Design review of the part built by this model. Coordinates are the model's own, in mm. Coordinates: 2 decimals unless noted, no trailing zeros. Order: outer loops, then holes, each group sorted by start corner. A loop starts at its lowest first (then second) coordinate and runs counter-clockwise, first axis right, second up. Notation, with made-up numbers: (35.5, -7.5) - (86.5, -7.5) arc R24 cw to (86.5, 12.5) - close; hole circle Ø8 at (87, 44). An arc over 180 degrees is marked (long way). Write item = value, one per line. Start each with the question number.
```python
from build123d import *

# Parameters (mm, degrees)
F1_DEPTH    = 3.175
F3_DEPTH    = 25.4
F4_T1_DEPTH = 21.629832931
F4_T3_DEPTH = 25.208081251
F6_D        = 3.175


# Not quite as in the source:
# - a fillet or chamfer that OpenCascade refuses, or shapes differently, is made with other operations: its cross-section is extruded or revolved along the edge and cut away or added


with BuildPart() as f1:
    # F0 (on Top) → F1 (new body, symmetric)
    with BuildSketch(Plane.XY):
        Polygon((-31.6706262529, 7.0008751936), (-31.4483754337, 0), (29.8926271498, 0), align=None)
    extrude(amount=F1_DEPTH, both=True)

    # F2 (on Front) → F3 (cut)
    with BuildSketch(Plane.XZ):
        Polygon((-32.3509715194, 5.2941306494), (-32.3509715194, 1.5875), (-19.0253787046, 1.5875), (-19.1175676882, 5.2941306494), align=None)
        Polygon((-19.0253787046, -1.5875), (-32.3509715194, -1.5875), (-32.3509715194, -5.2941306494), (-19.1175676882, -5.2941306494), align=None)
    extrude(amount=-F3_DEPTH, mode=Mode.SUBTRACT)

    # F4: fillet of radius 3.81 on 2 edges, made by hand

    # F4_s2 → F4_t1 (cut)
    with BuildSketch(Plane.XY.offset(-10.8149164655)):
        with BuildLine():
            ThreePointArc((-27.7574088475, 0), (-30.4083993967, 1.0735151913), (-31.5654904043, 3.6891080797))
            Line((-31.5654904043, 3.6891080797), (-31.4483754337, 0))
            Line((-31.4483754337, 0), (-27.7574088475, 0))
        make_face()
    extrude(amount=F4_T1_DEPTH, mode=Mode.SUBTRACT)

    # F4_s4 → F4_t3 (cut)
    with BuildSketch(Plane.XY.offset(-12.6040406255)):
        with BuildLine():
            ThreePointArc((-27.2922295058, 6.5029708841), (-30.3048140162, 5.5189587428), (-31.5308036019, 2.5964777998))
            Line((-31.5308036019, 2.5964777998), (-31.6706262529, 7.0008751936))
            Line((-31.6706262529, 7.0008751936), (-27.2922295058, 6.5029708841))
        make_face()
    extrude(amount=F4_T3_DEPTH, mode=Mode.SUBTRACT)

    # F6 (through all)
    with Locations(Plane(origin=(0, 0, -3.175), x_dir=(1, 0, 0), z_dir=(0, 0, -1))):
        with Locations((-27.722722045, -2.71736972)):
            Hole(F6_D / 2)


solid = f1.part
```
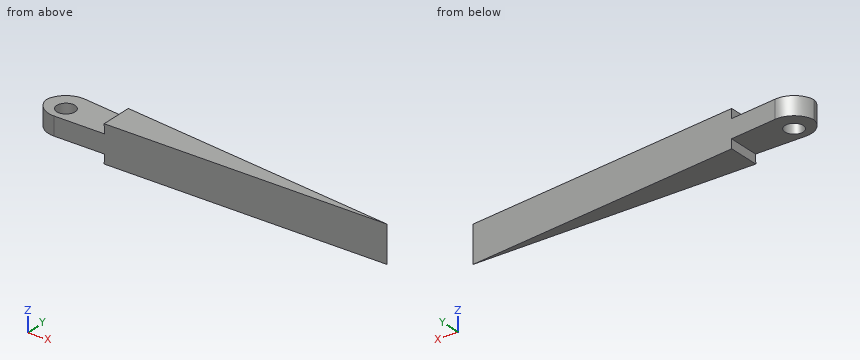
Item 1: Add section D-D on x = -3. Give the boundary of the cut face in (y, z) (1 decimal), plus the area to 3 significant figures.
Item 2: Add section B-B on y = 1.75. Give the boundary of the cut face in (x, z) (1 decimal), plus the area to 3 significant figures.
Item 3: For P1, Ø3.5, axis at x = -25, y = 4, coming from the -Z side; P2, Ø1, axis at x = -1.5, z = 0, coming from the +Y side; P3, Ø2, axis at y = 2.5, z = 0, coming from the -X side; P4, Ø3.5, axis at x = -24, y = 4, coming from the +Z side, all flat-tipped, find the tip position at first contact; note any pin that passes through.
Item 4: For line 1 (Z direction, x = -25.5, y = 2.5); line 2 (Y direction, x = -20, z = -1.25); line 3 (Y direction, x = -18, z = 2.5), list the stretches that pass through material, from the lowest coordinate up.
Item 5: Add section A-A on z = -0.75. Give the boundary of the cut face in (x, y) (1 decimal), plus the area to 3 significant figures.
Item 6: Add section C-C on y = 5. Give the boundary of the cut face in (x, z) (1 decimal), plus the area to 3 significant figures.
Worked out:
q1.outline = (0, -3.2) - (3.7, -3.2) - (3.7, 3.2) - (0, 3.2) - close
q1.area = 23.8 mm2
q2.outline = (-31, -1.6) - (-29, -1.6) - (-29, 1.6) - (-31, 1.6) - close; (-26.5, -1.6) - (-19, -1.6) - (-19.1, -3.2) - (14.5, -3.2) - (14.5, 3.2) - (-19.1, 3.2) - (-19, 1.6) - (-26.5, 1.6) - close
q2.area = 243 mm2
q3.P1 = -1.59
q3.P2 = 3.63
q3.P3 = -31.51
q3.P4 = 1.59
q4.line_1 = -1.59 to 1.59
q4.line_2 = 0 to 5.67
q4.line_3 = 0 to 5.45
q5.outline = (-31.5, 3.1) arc R3.8 ccw to (-27.8, 0) - (29.9, 0) - (-27.3, 6.5) arc R3.8 ccw to start; hole circle Ø3.2 at (-27.7, 2.7)
q5.area = 200 mm2
q6.outline = (-30.8, -1.6) - (-19, -1.6) - (-19.1, -3.2) - (-14.1, -3.2) - (-14.1, 3.2) - (-19.1, 3.2) - (-19, 1.6) - (-30.8, 1.6) - close
q6.area = 68.8 mm2
